```python
from build123d import *

# Parameters (mm, degrees)
SKETCH1_R           = 60
BOSS_EXTRUDE1_DEPTH = 16
SKETCH2_R           = 9
BOSS_EXTRUDE2_DEPTH = 220
FILLET1_R           = 6
FILLET2_R           = 1


with BuildPart() as part:
    # Sketch1 → Boss-Extrude1 (new body)
    with BuildSketch(Plane(origin=(0, 0, 0), x_dir=(1, 0, 0), z_dir=(0, 1, 0))):
        Circle(SKETCH1_R)
    extrude(amount=BOSS_EXTRUDE1_DEPTH)

    # Sketch2 → Boss-Extrude2 (add)
    with BuildSketch(Plane(origin=(0, 16, 0), x_dir=(1, 0, 0), z_dir=(0, 1, 0))):
        with Locations((0, 4.253298282)):
            Circle(SKETCH2_R)
    extrude(amount=BOSS_EXTRUDE2_DEPTH)

    # Fillet1
    fillet1_edges = [part.edges().sort_by_distance(p)[0] for p in [
        (-60, 16, 0),
    ]]
    fillet(fillet1_edges, radius=FILLET1_R)

    # Fillet2
    fillet2_edges = [part.edges().sort_by_distance(p)[0] for p in [
        (-60, 0, 0),
        (-9, 16, -4.253298282),
        (-9, 236, -4.253298282),
    ]]
    fillet(fillet2_edges, radius=FILLET2_R)


solid = part.part
```
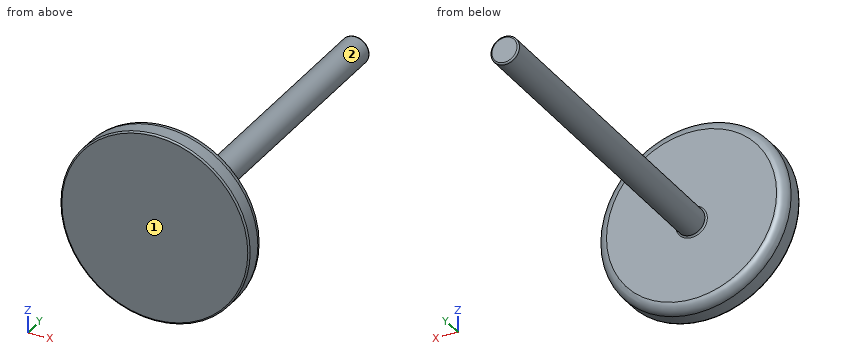
Can you work these out from the model? Positions are in its coordinate system, mm. Face numbers are marked on the shaded views. A direction names the side the tool comes from. Give positions to 0.01 mm unless a question says otherwise; leave off trailing zeros. Order: outer loops, then holes, each group sorted by start corner. A loop starts at its lowest first (then second) coordinate and runs counter-clockwise, first axis right, second up. Notation, with made-up numbers: M -7,31 L 0,31 A20 cw 0,52 Z; hole C -10.5,-34.5 d2. An arc over 180 degrees is marked long. Write item = value, one per line. Start each with the question number.
Q1. I need wall thicknesses on probe 1 along Y at (x, z) = (1.5, -40); probe 2 along Y at (x, z) = (-12, 53.5); probe 3 along X at (y, z) = (175, 1.5). Which ranges of each line are inside material? Lowest first, please. Write a range as [from, to].
Q2. For the marked faces 1 and 2, which set-ups out of +Z, -Z, +X, -X, +Y, -Y let a thin tool reach every point of the face, with its end or its side?
Q3. Suppose I cut it at B-B (y = 135.5). Write out the boundary of the cut face in (x, z), plus the area to 3 significant figures.
Q4. Will these pins go through, and if not, where does the flat tip stop? pin 1 Ø10 at (x, y) = (4, 167) entering from -Z; pin 2 Ø12 at (x, z) = (-6.5, 35) entering from +Y.
Q5. Suppose I cut it at A-A (x = 0). Write out the boundary of the cut face in (y, z).
Check result:
q1.probe_1 = [0, 16]
q1.probe_2 = [0, 15.94]
q1.probe_3 = [-6.92, 6.92]
q2.face_1 = +Z, -Z, +X, -X, -Y
q2.face_2 = +Y
q3.outline = C 0,-4.25 d18
q3.area = 254 mm2
q4.pin_1 = -13.25
q4.pin_2 = 16
q5.outline = M 0,-59 A1 ccw 1,-60 L 10,-60 A6 ccw 16,-54 L 16,-14.25 A1 cw 17,-13.25 L 235,-13.25 A1 ccw 236,-12.25 L 236,3.75 A1 ccw 235,4.75 L 17,4.75 A1 cw 16,5.75 L 16,54 A6 ccw 10,60 L 1,60 A1 ccw 0,59 Z
